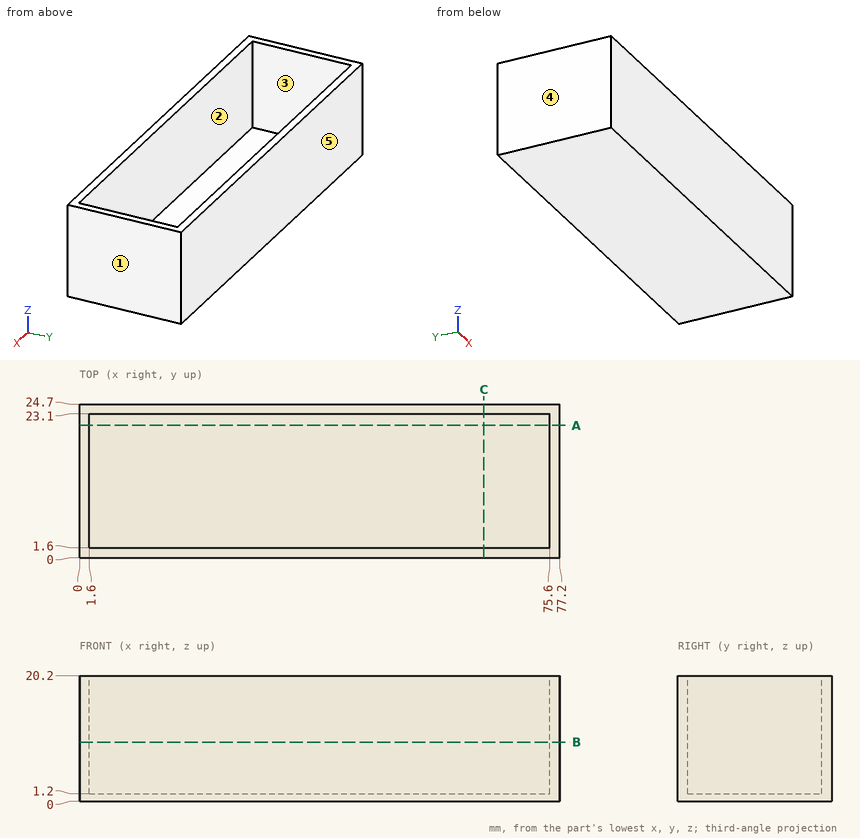
Geometry: see drawing. Coordinates: mm, zero at the bounding-box minimum. A direction names the side the tool comes from. Round coordinates to 2 decimals unless told otherwise and drop trailing zeros. Loops run counter-clockwise (first coordinate to the right, second up) from the corner with the lowest first, then second, coordinate; pieces in that order, holes last. Notation, with made-up numbers: (5, 88.25) -> (46, 88.25) arc R8 ccw to (46, 98.25) -> close; hole circle Ø11 at (43.25, 78.5). An arc over 180 degrees is marked (long way). One line per question, with ' | ' between items. Start each with the question number.
1. Section B-B on z = 9.5. Output: boundary loops of the cut face in (x, y).
2. Set-up query: the marked faces 1 and 2. Return all of +Z, -Z, +X, -X, +Y, -Y with unobstructed straight access to the full face (end or side cutting, diameter ignored); none if empty.
3. Mould query, pull axis X, two halves, no side actions, for the marked faces 3, 4 and 5. Classes: pulls with the +X half, pulls with the -X half, needs draft (parallel to the pull), parting line crosses it, or undercut.
4. Line query: line 1 along X through (y, z) = (8.75, 15.25); line 2 along Y through (x, z) = (60, 12.5); line 3 along Z through (x, y) = (30.5, 11). Output: solid intervals per line, ascending. Write a range as [from, to].
5. Contact query for a flat-ended pin moving along its axis: pin 1 (11 mm diameter, centred on x = 23, y = 8, fed in from +Z). Output: stop coordinate, or through.
6. Section A-A on y = 21.25. Output: boundary loops of the cut face in (x, z), and give its area (3 significant figures).
7. Section C-C on x = 65. Output: boundary loops of the cut face in (y, z), and give its area (3 significant figures).
Returned:
1) outline: (0, 0) -> (77.2, 0) -> (77.2, 24.7) -> (0, 24.7) -> close; hole (1.6, 1.6) -> (75.6, 1.6) -> (75.6, 23.1) -> (1.6, 23.1) -> close
2) face 1: +Z, -Z, +X, +Y, -Y | face 2: +Z
3) face 3: undercut | face 4: pulls with the -X half | face 5: needs draft
4) line 1: x = [0, 1.6], [75.6, 77.2] | line 2: y = [0, 1.6], [23.1, 24.7] | line 3: z = [0, 1.2]
5) pin 1: stops at z = 1.2
6) outline: (0, 0) -> (77.2, 0) -> (77.2, 20.2) -> (75.6, 20.2) -> (75.6, 1.2) -> (1.6, 1.2) -> (1.6, 20.2) -> (0, 20.2) -> close | area: 153 mm2
7) outline: (0, 0) -> (24.7, 0) -> (24.7, 20.2) -> (23.1, 20.2) -> (23.1, 1.2) -> (1.6, 1.2) -> (1.6, 20.2) -> (0, 20.2) -> close | area: 90.4 mm2
